Read the model definition and answer for the solid it produces. Units are mm, in the model's axes. A direction names the side the tool comes from. Coordinates: 2 decimals unless noted, no trailing zeros. Loops run counter-clockwise (first coordinate to the right, second up) from the corner with the lowest first, then second, coordinate; pieces in that order, holes last. Notation, with made-up numbers: (42, 77) -> (54, 77) arc R14 cw to (54, 104) -> close; hole circle Ø5 at (33.25, -33.75). An arc over 180 degrees is marked (long way). One line per question, with ' | ' between items. Start each with the question number.
```python
from build123d import *

# Parameters (mm, degrees)
F0_W     = 304.8
F0_H     = 38.1
F1_DEPTH = 63.5
F3_DEPTH = 127
F5_DEPTH = 38.1
F6_R     = 12.7
F7_DEPTH = 55.88
F9_DEPTH = 273.05


with BuildPart() as f1:
    # F0 (on Front) → F1 (new body, symmetric)
    with BuildSketch(Plane.XZ):
        with Locations((152.4, 19.05)):
            Rectangle(F0_W, F0_H)
    extrude(amount=F1_DEPTH, both=True)

    # F2 (on face) → F3 (join)
    with BuildSketch(Plane.XZ.offset(63.5)):
        Polygon((0, 82.55), (0, 38.1), (31.75, 38.1), (31.75, 101.6), (16.51, 101.6), align=None)
    extrude(amount=-F3_DEPTH)

    # F4 (on face) → F5 (join)
    with BuildSketch(Plane.YZ.offset(304.8)):
        with BuildLine():
            Line((-63.5, 50.8), (-63.5, 0))
            Line((-63.5, 0), (63.5, 0))
            Line((63.5, 0), (63.5, 50.8))
            Line((63.5, 50.8), (47.625, 50.8))
            Line((47.625, 50.8), (19.413296, 91.768501))
            ThreePointArc((19.413296, 91.768501), (-2.171038, 102.754075), (-23.151125, 90.654394))
            Line((-23.151125, 90.654394), (-47.625, 50.8))
            Line((-47.625, 50.8), (-63.5, 50.8))
        make_face()
    extrude(amount=-F5_DEPTH)

    # F6 (on face) → F7 (cut)
    with BuildSketch(Plane.YZ.offset(304.8)):
        with Locations((-1.506431, 77.362772)):
            Circle(F6_R)
    extrude(amount=-F7_DEPTH, mode=Mode.SUBTRACT)

    # F8 (on face) → F9 (cut)
    with BuildSketch(Plane.YZ.offset(304.8)):
        Polygon((-12.7, 0), (0, 0), (12.7, 0), (12.7, 16.51), (31.75, 16.51), (31.75, 29.21), (12.7, 29.21), (12.7, 38.1), (-12.7, 38.1), (-12.7, 29.21), (-31.75, 29.21), (-31.75, 16.51), (-12.7, 16.51), align=None)
    extrude(amount=-F9_DEPTH, mode=Mode.SUBTRACT)


solid = f1.part
```
(1) Each of these flat-tipped pins is pushed along its axis until it touches: pin 1 Ø10 at (y, z) = (-8, 55.5) entering from -X; pin 2 Ø4 at (x, y) = (123.5, -14.5) entering from +Z; pin 3 Ø17.5 at (x, y) = (292.5, 52.5) entering from +Z; pin 4 Ø1 at (y, z) = (-10.5, 12) entering from +X. Where does it stop, or does it pass through?
(2) Section D-D on y = -5 is taken. Write down the section's boundary in (x, z), plus the area to 3 significant figures.
(3) Section B-B on x = 148 is taken. Write down the section's boundary in (y, z), plus the area to 3 significant figures.
(4) Find the intervals of material crossed by probe 1 along X at (y, z) = (10.5, 69); probe 2 along Z at (x, y) = (181, -26.5); probe 3 along Z at (x, y) = (64.5, -41.5), in increasing order. Write a range as from..to.
(5) A tool of negligible diameter and unlimited length cuts with its end or side. For faces 4 (the flat face through (170, 22, 16.51)), 5 (the flat face through (266.7, -1, 64)), 6 (the flat face through (286.017, 33.717, 70.997)), 7 (the cylindrical face through (286.02, -1.82, 102.76)), from which of +Z, -Z, +X, -X, +Y, -Y can it reach the whole face along a straight path? Write none if from no direction.
(6) Section A-A on z = 42 is taken. Write down the section's boundary in (x, y).
(7) Determine the mould class of faces 1 (the flat face through (286, -55, 50.8)), 2 (the flat face through (148, -38, 38.1)), 3 (the flat face through (0, -1, 42)) for opening direction X: +X half, -X half, draft (parallel to the pull), parting line (faces both ways), or undercut.
Working result:
1) pin 1: stops at x = 0 | pin 2: stops at z = 38.1 | pin 3: stops at z = 56.43 | pin 4: stops at x = 31.75
2) outline: (0, 0) -> (31.75, 0) -> (31.75, 101.6) -> (16.51, 101.6) -> (0, 82.55) -> close; (266.7, 38.1) -> (304.8, 38.1) -> (304.8, 65.15) -> (266.7, 65.15) -> close; (266.7, 89.57) -> (304.8, 89.57) -> (304.8, 102.52) -> (266.7, 102.52) -> close | area: 4,590 mm2
3) outline: (-63.5, 0) -> (-12.7, 0) -> (-12.7, 16.51) -> (-31.75, 16.51) -> (-31.75, 29.21) -> (-12.7, 29.21) -> (-12.7, 38.1) -> (-63.5, 38.1) -> close; (12.7, 0) -> (63.5, 0) -> (63.5, 38.1) -> (12.7, 38.1) -> (12.7, 29.21) -> (31.75, 29.21) -> (31.75, 16.51) -> (12.7, 16.51) -> close | area: 3,390 mm2
4) probe 1: x = 0..31.75, 266.7..304.8 | probe 2: z = 0..16.51, 29.21..38.1 | probe 3: z = 0..38.1
5) face 4: +X | face 5: +Z, +Y, -Y | face 6: +Z, +X, +Y | face 7: +Z, +X
6) outline: (0, -63.5) -> (31.75, -63.5) -> (31.75, 63.5) -> (0, 63.5) -> close; (266.7, -63.5) -> (304.8, -63.5) -> (304.8, 63.5) -> (266.7, 63.5) -> close
7) face 1: draft | face 2: undercut | face 3: -X half
